The figure shows three views and two pictorial views of one solid part (mm, origin at its lowest corner). Answer the questions. A direction names the side the tool comes from. Coordinates: 2 decimals unless noted, no trailing zeros. Write each loop counter-clockwise with the first axis right and the second up, starting at its lowest first coordinate (ties: lowest second). Pieces come first, ordered by that corner, then holes. Notation, with made-up numbers: M 35,-10.75 L 65,-10.75 A13 ccw 65,10.25 Z; hole C 70.5,1.25 d8. An arc over 180 degrees is marked long. Write item = value, one per line.
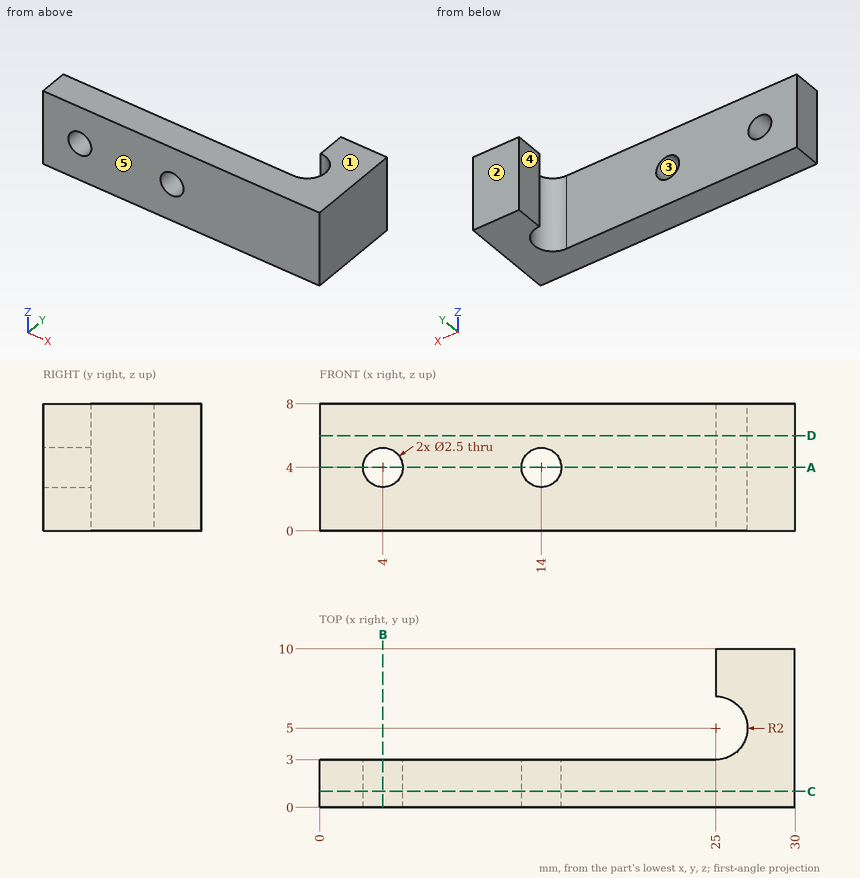
Item 1: Flat-ended cylindrical pins translate along their axes: pin 1 (2 mm diameter, centred on x = 25.5, z = 3, fed in from -Y); pin 2 (0.9 mm diameter, centred on y = 8.5, z = 2, fed in from -X); pin 3 (2 mm diameter, centred on x = 14.5, z = 5.5, fed in from +Y). Find the tip coordinate at first contact, or state that the pin passes through.
Worked answers:
pin_1 = 0
pin_2 = 25
pin_3 = 3
Item 2: For a pull along Z with two mould halves and no side action, classify the marked faces 1, 2 and 3 as released by +Z, released by -Z, zero draft, split by the parting line, or undercut.
Worked answers:
face_1 = released by +Z
face_2 = zero draft
face_3 = undercut
Item 3: Find section D-D (z = 6). Determine the outline of the cut face in (x, y), and give its area (3 significant figures).
Worked answers:
outline = M 0,0 L 30,0 L 30,10 L 25,10 L 25,7 A2 cw 25,3 L 0,3 Z
area = 119 mm²
Item 4: Find section A-A (z = 4). Determine the outline of the cut face in (x, y), and give its area (3 significant figures).
Worked answers:
outline = M 0,0 L 2.75,0 L 2.75,3 L 0,3 Z; M 5.25,0 L 12.75,0 L 12.75,3 L 5.25,3 Z; M 15.25,0 L 30,0 L 30,10 L 25,10 L 25,7 A2 cw 25,3 L 15.25,3 Z
area = 104 mm²
Item 5: Consider line 1 along X through (y, z) = (2, 4); line 2 along Z through (x, y) = (14, 0.9); line 3 along X through (y, z) = (2.5, 3). Determine where each line is inside the solid, lowest interval first. Write a range as from..to.
Worked answers:
line_1 = 0..2.75, 5.25..12.75, 15.25..30
line_2 = 0..2.75, 5.25..8
line_3 = 0..3.25, 4.75..13.25, 14.75..30
Item 6: Find section C-C (y = 1). Determine the outline of the cut face in (x, z), and give its area (3 significant figures).
Worked answers:
outline = M 0,0 L 30,0 L 30,8 L 0,8 Z; hole C 4,4 d2.5; hole C 14,4 d2.5
area = 230 mm²
Item 7: Which of the six approach directions +Z, -Z, +X, -X, +Y, -Y give full straight-line access (tool end or side, diameter ignored) to the marked faces 4 and 5?
Worked answers:
face_4 = +Z, -Z, -X, +Y
face_5 = +Z, -Z, +X, -X, -Y
Item 8: Find section B-B (x = 4). Determine the outline of the cut face in (y, z).
Worked answers:
outline = M 0,0 L 3,0 L 3,2.75 L 0,2.75 Z; M 0,5.25 L 3,5.25 L 3,8 L 0,8 Z
